The listing builds one solid part. Answer for the finished solid, in the listing's coordinates (mm). Face numbers are marked on the shaded views. A direction names the side the tool comes from. Round coordinates to 2 decimals unless told otherwise and drop trailing zeros. Write each loop counter-clockwise with the first axis right and the second up, starting at its lowest first coordinate (ties: lowest second). Pieces come first, ordered by that corner, then holes.
Item 1: Find section A-A on y = -11. Give the vertices of the cut face in (x, z).
Item 2: For a pull along X with two mould halves and no side action, classify the marked faces 1, 2 and 3 as +X half, -X half, draft (parallel to the pull), parting line (faces both ways), or undercut.
Item 3: Find section C-C on y = -22. Give the vertices of the cut face in (x, z), then the cut area to 3 significant figures.
Item 4: Each of these flat-tipped pins is pushed along its axis until it touches: pin 1 (3 mm diameter, centred on x = 11, y = -9.5, fed in from +Z); pin 2 (1.5 mm diameter, centred on x = 9, y = -17.5, fed in from -Z); pin 3 (6.5 mm diameter, centred on x = 6, y = -25, fed in from -Z). Where does it stop, or does it pass through?
Item 5: A tool of negligible diameter and unlimited length cuts with its end or side. For the marked faces 4, 5, 6 and 7, from which of +Z, -Z, +X, -X, +Y, -Y can it reach the whole face along a straight path? Write none if from no direction.
Item 6: Find section D-D on x = 7.5. Give the vertices of the cut face in (y, z), then the cut area to 3 significant figures.
Item 7: Find section B-B on x = 0. Give the vertices of the cut face in (y, z), then the cut area to 3 significant figures.
Item 8: Find the intervals of material crossed by probe 1 along Y at (x, z) = (-0.5, 1.25); probe 2 along X at (y, z) = (-11, 1.75); probe 3 along Y at (x, z) = (0, 3.3), in increasing order.
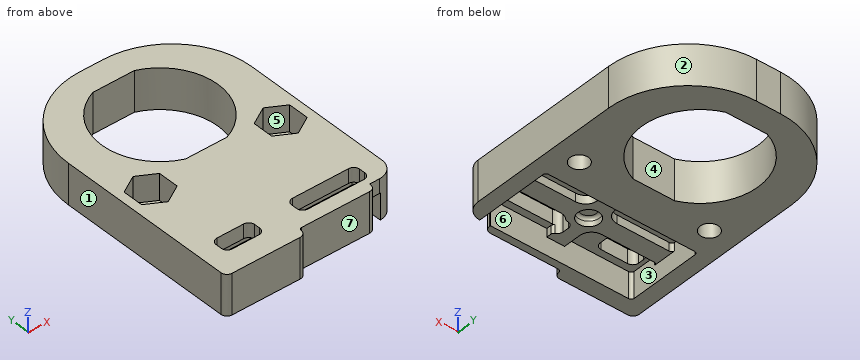
```python
from build123d import *

# Parameters (mm, degrees)
SKETCH_R        = 1.55
SKETCH_W        = 6.5
SKETCH_H        = 3
SKETCH_W_2      = 11.5
PAD_DEPTH       = 6.8
SKETCH005_W     = 25.7
SKETCH005_H     = 13
POCKET_DEPTH    = 3
SKETCH006_R     = 1.8
POCKET001_DEPTH = 1.4
POCKET002_DEPTH = 4.4
FILLET_R        = 1
FILLET001_R     = 0.5


with BuildPart() as part:
    # Sketch → Pad (new body)
    with BuildSketch(Plane.XY):
        with BuildLine():
            Line((-2, 13.5), (2, 13.5))
            ThreePointArc((15.5, 0), (11.545942, 9.545942), (2, 13.5))
            Line((15.5, 0), (15.5, -25.7))
            ThreePointArc((12.7, -28.5), (14.679899, -27.679899), (15.5, -25.7))
            Line((11.04, -28.5), (12.7, -28.5))
            Line((11.04, -29.7), (11.04, -28.5))
            Line((-1.96, -29.7), (11.04, -29.7))
            Line((-1.96, -31.15), (-1.96, -29.7))
            Line((-1.96, -31.15), (-15.5, -31.15))
            Line((-15.5, -31.15), (-15.5, 0))
            ThreePointArc((-2, 13.5), (-11.545942, 9.545942), (-15.5, 0))
        make_face()
        with Locations((-11, -11)):
            Circle(SKETCH_R, mode=Mode.SUBTRACT)
        with Locations((11, -11)):
            Circle(SKETCH_R, mode=Mode.SUBTRACT)
        with BuildLine():
            ThreePointArc((-3.50963, 9.15), (-9.8, 0), (-3.50963, -9.15))
            Line((3.50963, -9.15), (-3.50963, -9.15))
            ThreePointArc((3.50963, -9.15), (9.8, 0), (3.50963, 9.15))
            Line((-3.50963, 9.15), (3.50963, 9.15))
        make_face(mode=Mode.SUBTRACT)
        with Locations((-8.91, -25.81)):
            Rectangle(SKETCH_W, SKETCH_H, mode=Mode.SUBTRACT)
        with Locations((6.35, -25.81)):
            Rectangle(SKETCH_W_2, SKETCH_H, mode=Mode.SUBTRACT)
    extrude(amount=PAD_DEPTH)

    # Sketch005 (on Face26 of Pad) → Pocket (cut)
    with BuildSketch(Plane(origin=(0, 0, 0), x_dir=(1, 0, 0), z_dir=(0, 0, -1))):
        with Locations((0, 22)):
            Rectangle(SKETCH005_W, SKETCH005_H)
    extrude(amount=-POCKET_DEPTH, mode=Mode.SUBTRACT)

    # Sketch006 (on Face32 of Pocket) → Pocket001 (cut)
    with BuildSketch(Plane(origin=(0, 0, 3), x_dir=(1, 0, 0), z_dir=(0, 0, -1))):
        with Locations((0, 22)):
            Circle(SKETCH006_R)
        with BuildLine():
            Line((-12.85, 20.5), (-3.5, 20.5))
            ThreePointArc((-1.5, 18.5), (-2.085786, 19.914214), (-3.5, 20.5))
            Line((-1.5, 18.5), (-1.5, 15.5))
            Line((-1.5, 15.5), (-12.85, 15.5))
            Line((-12.85, 15.5), (-12.85, 20.5))
        make_face()
        with BuildLine():
            Line((1.5, 15.5), (12.85, 15.5))
            Line((12.85, 15.5), (12.85, 20.5))
            Line((12.85, 20.5), (3.5, 20.5))
            ThreePointArc((3.5, 20.5), (2.085786, 19.914214), (1.5, 18.5))
            Line((1.5, 18.5), (1.5, 15.5))
        make_face()
        with BuildLine():
            Line((-12.85, 23.5), (-3.5, 23.5))
            ThreePointArc((-3.5, 23.5), (-2.085786, 24.085786), (-1.5, 25.5))
            Line((-1.5, 25.5), (-1.5, 28.5))
            Line((-1.5, 28.5), (-12.85, 28.5))
            Line((-12.85, 28.5), (-12.85, 23.5))
        make_face()
        with BuildLine():
            Line((1.5, 28.5), (12.85, 28.5))
            Line((12.85, 28.5), (12.85, 23.5))
            Line((12.85, 23.5), (3.5, 23.5))
            ThreePointArc((1.5, 25.5), (2.085786, 24.085786), (3.5, 23.5))
            Line((1.5, 25.5), (1.5, 28.5))
        make_face()
    extrude(amount=-POCKET001_DEPTH, mode=Mode.SUBTRACT)

    # Sketch001 (on Face5 of Pocket001) → Pocket002 (cut)
    with BuildSketch(Plane.XY.offset(6.8)):
        Polygon((-8, -12.732051), (-8, -9.267949), (-11, -7.535898), (-14, -9.267949), (-14, -12.732051), (-11, -14.464102), align=None)
        Polygon((14, -12.732051), (14, -9.267949), (11, -7.535898), (8, -9.267949), (8, -12.732051), (11, -14.464102), align=None)
    extrude(amount=-POCKET002_DEPTH, mode=Mode.SUBTRACT)

    # Fillet
    fillet_edges = [part.edges().sort_by_distance(p)[0] for p in [
        (-15.5, -31.15, 3.4),
        (-1.96, -31.15, 3.4),
        (11.04, -29.7, 3.4),
        (0.6, -24.31, 4.9),
        (-12.16, -24.31, 5.6),
        (-12.16, -27.31, 5.6),
        (0.6, -27.31, 4.9),
        (-5.66, -24.31, 5.6),
        (12.1, -24.31, 5.6),
        (-5.66, -27.31, 5.6),
        (12.1, -27.31, 5.6),
    ]]
    fillet(fillet_edges, radius=FILLET_R)

    # Fillet001
    fillet001_edges = [part.edges().sort_by_distance(p)[0] for p in [
        (12.85, -15.5, 1.5),
        (12.85, -15.5, 3.7),
        (12.85, -20.5, 3.7),
        (-12.85, -20.5, 3.7),
        (12.85, -23.5, 3.7),
        (-12.85, -23.5, 3.7),
        (-12.85, -15.5, 3.7),
        (-12.85, -15.5, 1.5),
        (-12.85, -28.5, 3.7),
        (-12.85, -28.5, 1.5),
        (1.5, -27.304987, 3.7),
        (-1.96, -29.7, 3.4),
        (-1.8, -22, 4.4),
        (1.892549, -24.31, 3.7),
    ]]
    fillet(fillet001_edges, radius=FILLET001_R)


solid = part.part
```
Check values:
1. outline: (-15.5, 0) - (-12.55, 0) - (-12.55, 2.4) - (-14, 2.4) - (-14, 6.8) - (-15.5, 6.8) - close; (-9.45, 0) - (9.45, 0) - (9.45, 2.4) - (8, 2.4) - (8, 6.8) - (-8, 6.8) - (-8, 2.4) - (-9.45, 2.4) - close; (12.55, 0) - (15.5, 0) - (15.5, 6.8) - (14, 6.8) - (14, 2.4) - (12.55, 2.4) - close
2. face 1: -X half
2. face 2: +X half
2. face 3: undercut
3. outline: (-15.5, 0) - (-12.85, 0) - (-12.85, 3) - (-1.8, 3) - (-1.8, 3.9) arc R0.5 cw to (-1.3, 4.4) - (1.3, 4.4) arc R0.5 cw to (1.8, 3.9) - (1.8, 3) - (12.85, 3) - (12.85, 0) - (15.5, 0) - (15.5, 6.8) - (-15.5, 6.8) - close
3. area: 129 mm2
4. pin 1: stops at z = 2.4
4. pin 2: stops at z = 4.4
4. pin 3: stops at z = 3
5. face 4: +Z, -Z
5. face 5: +Z
5. face 6: -Z
5. face 7: +Z, -Z, +X, -Y
6. outline: (-29.7, 0) - (-28.5, 0) - (-28.5, 4.4) - (-27.31, 4.4) - (-27.31, 6.8) - (-29.7, 6.8) - close; (-24.31, 4.4) - (-23.5, 4.4) - (-23.5, 3) - (-20.5, 3) - (-20.5, 4.4) - (-15.5, 4.4) - (-15.5, 0) - (-6.31, 0) - (-6.31, 6.8) - (-24.31, 6.8) - close; (6.31, 0) - (12.33, 0) - (12.33, 6.8) - (6.31, 6.8) - close
6. area: 140 mm2
7. outline: (-29.7, 0) - (-28.5, 0) - (-28.5, 3) - (-23.8, 3) - (-23.8, 3.9) arc R0.5 cw to (-23.3, 4.4) - (-20.7, 4.4) arc R0.5 cw to (-20.2, 3.9) - (-20.2, 3) - (-15.5, 3) - (-15.5, 0) - (-9.15, 0) - (-9.15, 6.8) - (-29.7, 6.8) - close; (9.15, 0) - (13.5, 0) - (13.5, 6.8) - (9.15, 6.8) - close
7. area: 125 mm2
8. probe 1: y = -29.7 to -28.5, -15.5 to -9.15, 9.15 to 13.5
8. probe 2: x = -15.5 to -12.55, -9.45 to 9.45, 12.55 to 15.5
8. probe 3: y = -29.7 to -23.8, -20.2 to -9.15, 9.15 to 13.5
